Part model, mm, in its own coordinate system. Round coordinates to 2 decimals unless told otherwise and drop trailing zeros. Write each loop counter-clockwise with the first axis right and the second up, starting at its lowest first coordinate (ties: lowest second). Pieces come first, ordered by that corner, then holes.
1) Saw through at A-A on y = -80.5. Write the cut outline in (x, z).
2) Drill centre lines: L1, parallel to Y at x = -152.5, z = 0.9; L2, parallel to Y at x = -133.6, z = 0.15; L3, parallel to Y at x = 6, z = 1.25. Where is each one in solid material? Low to high.
3) Saw through at C-C on z = -0.45. Count the separate pieces of the cut face and the enclosed holes in it, and give its area (3 significant figures).
4) Saw through at B-B on x = -99. Write the cut outline in (y, z), and give its area (3 significant figures).
5) Flat gauge pin, fed straight in: pin 1 (6 mm diameter, centred on x = 230, y = 154.12, fed in from -Z). Where does the tip first touch, or does it go through?
```python
from build123d import *

# Parameters (mm, degrees)
SKETCH1_W            = 492
SKETCH1_H            = 515.3
BOSS_EXTRUDE1_DEPTH  = 1.5
M6_CLEARANCE_HOLE1_D = 6.6
M6_CLEARANCE_HOLE2_D = 6.6
FILLET1_R            = 35
CUT_EXTRUDE1_DEPTH   = 357.242224477
M4_CLEARANCE_HOLE1_D = 4.5
M4_CLEARANCE_HOLE2_D = 4.5


with BuildPart() as part:
    # Sketch1 → Boss-Extrude1 (new, symmetric)
    with BuildSketch(Plane.XY):
        Rectangle(SKETCH1_W, SKETCH1_H)
    extrude(amount=BOSS_EXTRUDE1_DEPTH, both=True)

    # M6 Clearance Hole1 (through all)
    with Locations(Plane(origin=(0, 0, -1.5), x_dir=(-1, 0, 0), z_dir=(0, 0, -1))):
        with Locations((-230, 154.116994756), (-230, 124.116994756), (-230, 94.116994756), (-230, -94.116994756), (-230, -124.116994756), (-230, -154.116994756)):
            Hole(M6_CLEARANCE_HOLE1_D / 2)

    # M6 Clearance Hole2 (through all)
    with Locations(Plane(origin=(0, 0, -1.5), x_dir=(-1, 0, 0), z_dir=(0, 0, -1))):
        with Locations((211, 25), (211, -25), (186, 0)):
            Hole(M6_CLEARANCE_HOLE2_D / 2)

    # Fillet1
    fillet1_edges = [part.edges().sort_by_distance(p)[0] for p in [
        (246, -257.65, 0),
        (-246, -257.65, 0),
        (-246, 257.65, 0),
        (246, 257.65, 0),
    ]]
    fillet(fillet1_edges, radius=FILLET1_R)

    # Sketch6 → Cut-Extrude1 (cut, through all)
    with BuildSketch(Plane(origin=(0, 0, -1.5), x_dir=(-1, 0, 0), z_dir=(0, 0, -1))):
        with BuildLine():
            Line((-133.5, -100), (133.5, -100))
            ThreePointArc((133.5, -100), (140.571067812, -97.071067812), (143.5, -90))
            Line((143.5, -90), (143.5, 90))
            ThreePointArc((143.5, 90), (140.571067812, 97.071067812), (133.5, 100))
            Line((133.5, 100), (-133.5, 100))
            ThreePointArc((-133.5, 100), (-140.571067812, 97.071067812), (-143.5, 90))
            Line((-143.5, 90), (-143.5, -90))
            ThreePointArc((-143.5, -90), (-140.571067812, -97.071067812), (-133.5, -100))
        make_face()
    extrude(amount=-CUT_EXTRUDE1_DEPTH, mode=Mode.SUBTRACT)

    # M4 Clearance Hole1 (through all)
    with Locations(Plane(origin=(0, 0, -1.5), x_dir=(-1, 0, 0), z_dir=(0, 0, -1))):
        with Locations((-133.6, -109), (-66.8, -109), (0, -109), (66.8, -109), (133.6, -109), (152.5, -90.1), (152.5, -45.05), (152.5, 0), (152.5, 45.05), (152.5, 90.1), (133.6, 109), (66.8, 109), (0, 109), (-66.8, 109), (-133.6, 109), (-152.5, 90.1), (-152.5, 45.05), (-152.5, 0), (-152.5, -45.05), (-152.5, -90.1)):
            Hole(M4_CLEARANCE_HOLE1_D / 2)

    # M4 Clearance Hole2 (through all)
    with Locations(Plane(origin=(0, 0, -1.5), x_dir=(-1, 0, 0), z_dir=(0, 0, -1))):
        with Locations((226.4, 194.65), (226.4, 172.65)):
            Hole(M4_CLEARANCE_HOLE2_D / 2)


solid = part.part
```
Completed:
1. outline: (-246, -1.5) - (-143.5, -1.5) - (-143.5, 1.5) - (-246, 1.5) - close; (143.5, -1.5) - (246, -1.5) - (246, 1.5) - (143.5, 1.5) - close
2. L1: y = -257.65 to -92.35, -87.85 to -47.3, -42.8 to -2.25, 2.25 to 42.8, 47.3 to 87.85, 92.35 to 257.65
2. L2: y = -257.65 to -111.25, -106.75 to -100, 100 to 106.75, 111.25 to 257.65
2. L3: y = -257.65 to -100, 100 to 257.65
3. separate pieces: 1
3. enclosed holes: 32
3. area: 195,000 mm2
4. outline: (-257.65, -1.5) - (-100, -1.5) - (-100, 1.5) - (-257.65, 1.5) - close; (100, -1.5) - (257.65, -1.5) - (257.65, 1.5) - (100, 1.5) - close
4. area: 946 mm2
5. pin 1: passes through
